CAD build for the part. Positions are in the model's coordinates, mm. Face numbers are marked on the shaded views. A direction names the side the tool comes from. Give positions to 0.01 mm unless a question says otherwise; leave off trailing zeros. Loops run counter-clockwise (first coordinate to the right, second up) from the corner with the lowest first, then second, coordinate; pieces in that order, holes last. Notation, with made-up numbers: (88.5, -19) -> (108.5, -19) arc R10 ccw to (108.5, -15) -> close; hole circle Ø7 at (-30.5, 57). An arc over 180 degrees is marked (long way). Use one line per item in the form item = value.
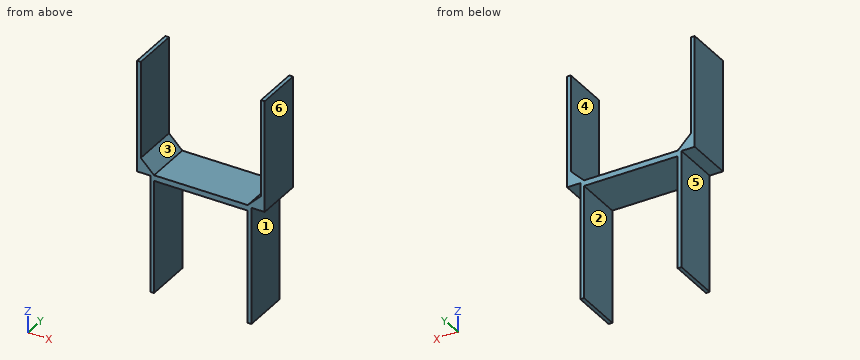
```python
from build123d import *

# Parameters (mm, degrees)
BOSS_EXTRU_1_DEPTH = 25
BOSS_EXTRU_2_DEPTH = 2
BOSS_EXTRU_3_DEPTH = 2
BOSS_EXTRU_5_DEPTH = 2
ESQUISSE4_W        = 12.5
ESQUISSE4_H        = 25
BOSS_EXTRU_6_DEPTH = 2


with BuildPart() as part:
    # Esquisse1 → Boss.-Extru.1 (new body)
    with BuildSketch(Plane(origin=(0, 0, 0), x_dir=(1, 0, 0), z_dir=(0, 1, 0))):
        Polygon((-34.071067812, -19.102794325), (-34.071067812, -12.031726513), (-27, -12.031726513), (-27, 37.968273487), (-25, 37.968273487), (-25, -9.860153638), (25, -9.860153638), (25, 37.968273487), (27, 37.968273487), (27, -12.031726513), (34.071067812, -12.031726513), (34.071067812, -19.102794325), (34.071067812, -59.102794325), (32.071067812, -59.102794325), (32.071067812, -19.93122145), (25, -12.860153638), (-25, -12.860153638), (-32.071067812, -19.93122145), (-32.071067812, -59.102794325), (-34.071067812, -59.102794325), align=None)
    extrude(amount=BOSS_EXTRU_1_DEPTH)

    # Esquisse2 → Boss.-Extru.2 (add)
    with BuildSketch(Plane(origin=(34.071067812, 0, 0), x_dir=(0, 0, -1), z_dir=(1, 0, 0))):
        Polygon((-59.102794325, 25), (-71.602794325, 25), (-71.602794325, 0), (-59.102794325, 0), (-12.031726513, 0), (-12.031726513, 25), align=None)
    extrude(amount=-BOSS_EXTRU_2_DEPTH)

    # Esquisse3 → Boss.-Extru.3 (add)
    with BuildSketch(Plane(origin=(27, 0, 0), x_dir=(0, 0, -1), z_dir=(1, 0, 0))):
        Polygon((37.947300388, 25), (50.447300388, 25), (50.491690046, 0), (37.947300388, 0), align=None)
    extrude(amount=-BOSS_EXTRU_3_DEPTH)

    # Esquisse5 → Boss.-Extru.5 (add)
    with BuildSketch(Plane.ZY.offset(27)):
        Polygon((-37.968273487, 0), (-37.968273487, 25), (-50.447300388, 25), (-50.491690046, 0), align=None)
    extrude(amount=-BOSS_EXTRU_5_DEPTH)

    # Esquisse4 → Boss.-Extru.6 (add)
    with BuildSketch(Plane.ZY.offset(34.071067812)):
        with Locations((65.352794325, 12.5)):
            Rectangle(ESQUISSE4_W, ESQUISSE4_H)
    extrude(amount=-BOSS_EXTRU_6_DEPTH)


solid = part.part
```
1. Cut at D-D, the plane x = -1. Write the cut outline in (y, z), then the cut area to 3 significant figures.
Result sheet:
outline = (0, 9.86) -> (25, 9.86) -> (25, 12.86) -> (0, 12.86) -> close
area = 75.0 mm^2
2. Cut at B-B, the plane y = 11.25. Write the cut outline in (x, z), then the cut area to 3 significant figures.
Result sheet:
outline = (-34.07, 12.03) -> (-27, 12.03) -> (-27, -50.47) -> (-25, -50.47) -> (-25, 9.86) -> (25, 9.86) -> (25, -50.47) -> (27, -50.47) -> (27, 12.03) -> (34.07, 12.03) -> (34.07, 71.6) -> (32.07, 71.6) -> (32.07, 19.93) -> (25, 12.86) -> (-25, 12.86) -> (-32.07, 19.93) -> (-32.07, 71.6) -> (-34.07, 71.6) -> close
area = 700 mm^2
3. Cut at A-A, the plane z = -4.5. Write the cut outline in (x, y).
Result sheet:
outline = (-27, 0) -> (-25, 0) -> (-25, 25) -> (-27, 25) -> close; (25, 0) -> (27, 0) -> (27, 25) -> (25, 25) -> close
4. Mould opens along X. For the marked faces 4, 5 and 6 say: pulls with the +X half, pulls with the -X half, needs draft (parallel to the pull), parting line crosses it, or undercut.
Result sheet:
face_4 = undercut
face_5 = pulls with the -X half
face_6 = pulls with the +X half
5. Cut at C-C, the plane z = 17. Write the cut outline in (x, y).
Result sheet:
outline = (-34.07, 0) -> (-29.14, 0) -> (-29.14, 25) -> (-34.07, 25) -> close; (29.14, 0) -> (34.07, 0) -> (34.07, 25) -> (29.14, 25) -> close
6. Tool access for the marked faces 1, 2 and 3: list every direction of +Z, -Z, +X, -X, +Y, -Y with a clear straight run to the whole face (end or side of a thin tool).
Result sheet:
face_1 = -Z, +X, +Y, -Y
face_2 = -Z, +Y, -Y
face_3 = +Z, +Y, -Y
7. Drop flat-ended pins along their axis: P1, Ø8, axis at x = -4.5, y = 18.5, coming from the +Z side; P2, Ø10, axis at x = -18.5, z = 16, coming from the +Y side; P3, Ø7.5, axis at y = 17, z = -17, coming from the +X side; P4, Ø5.5, axis at x = 31, y = 9.5, coming from the -Z side. Give the stop position or say it passes through.
Result sheet:
P1 = 12.86
P2 = 25
P3 = 27
P4 = 12.03
8. Drill centre lines: line 1 (X direction, y = 16, z = 25); line 2 (X direction, y = 18.75, z = -10.5); line 3 (Z direction, x = 7.5, y = 17.5). Where is each one in solid material? Low to high.
Result sheet:
line_1 = -34.07 to -32.07, 32.07 to 34.07
line_2 = -27 to -25, 25 to 27
line_3 = 9.86 to 12.86
